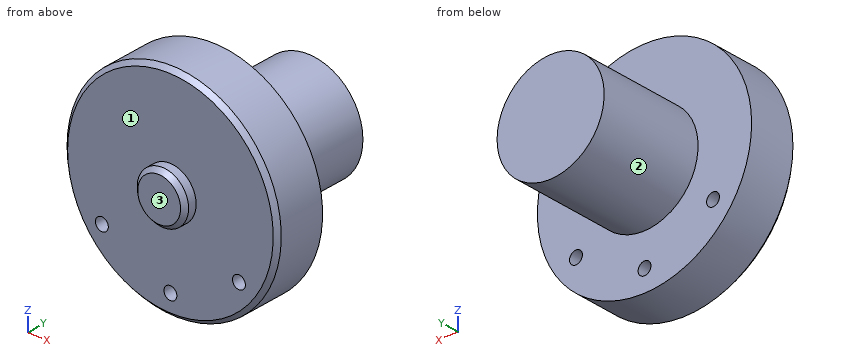
Autodesk Inventor part; units mm, degrees
ref_plane "YZ Plane" through (0, 0, 0) normal (1, 0, 0) x (0, 1, 0)
ref_plane "XZ Plane" through (0, 0, 0) normal (0, 1, 0) x (-1, 0, 0)
ref_plane "XY Plane" through (0, 0, 0) normal (0, 0, 1) x (1, 0, 0)
sketch "Szkic1" plane through (0, 0, 0) normal (0, 1, 0) x (-1, 0, 0)
  circle A0 centre (0, 0) radius 25
  dimension "d0" = 50
extrude "Wyciągnięcie proste1" add sketch "Szkic1" along normal blind 12
sketch "Szkic2" plane through (0, 0, 0) normal (0, -1, 0) x (1, 0, 0)
  circle A0 centre (0, 0) radius 6
  dimension "d3" = 12
extrude "Wyciągnięcie proste2" add sketch "Szkic2" along normal blind 3
sketch "Szkic3" plane through (0, 12, 0) normal (0, 1, 0) x (1, 0, 0)
  circle A0 centre (0, 0) radius 12.5
  dimension "d6" = 25
extrude "Wyciągnięcie proste3" add sketch "Szkic3" along normal blind 25
chamfer "Faza1" distance 1 angle 45 1 edges at (-6, -3, 0)
chamfer "Faza2" distance 1 angle 45 1 edges at (25, 0, 0)
sketch "Szkic6" plane through (0, 0, 0) normal (0, -1, 0) x (1, 0, 0)
  circle A0 centre (0, 0) radius 20
  circle A1 centre (-16, -12) radius 1.5
  dimension "d16" = 40
  dimension "d17" = 3
extrude "Wyciągnięcie proste4" cut sketch "Szkic6" against normal blind 25 contours A1 A0 | A0 A1 picked at (-15.6226, -11.6657) picked at (-16.3566, -12.3446)
sketch "Szkic7" plane through (0, 0, 0) normal (0, -1, 0) x (1, 0, 0)
  circle A0 centre (0, 0) radius 5
  circle A1 centre (0, 0) radius 20
  circle A2 centre (16, -12) radius 1.5
  dimension "d20" = 40
  dimension "d21" = 3
extrude "Wyciągnięcie proste5" cut sketch "Szkic7" against normal blind 25 contours A2 A1 | A1 A2 picked at (15.5641, -11.7467) picked at (16.3868, -12.3102)
sketch "Szkic9" plane through (0, 0, 0) normal (0, -1, 0) x (1, 0, 0)
  circle A0 centre (0, -20) radius 1.5
  point P0 (0, 0)
  dimension "d25" = 3
extrude "Wyciągnięcie proste6" cut sketch "Szkic9" against normal blind 25
The listing builds one solid part. Answer for the finished solid, in the listing's coordinates (mm). Face numbers are marked on the shaded views. A direction names the side the tool comes from. Round coordinates to 2 decimals unless told otherwise and drop trailing zeros. Loops run counter-clockwise (first coordinate to the right, second up) from the corner with the lowest first, then second, coordinate; pieces in that order, holes last.
Q1. Given pin 1 Ø10 at (x, z) = (10, -16.5) entering from +Y; pin 2 Ø24 at (x, z) = (-5.5, -9.5) entering from -Y; pin 3 Ø8 at (x, y) = (-10, 22.5) entering from -Z; pin 4 Ø3 at (x, z) = (-1.5, -8) entering from -Y, each flat-ended and moving along its own axis, determine where each tip first touches the part or whether it passes through.
Q2. Find the intervals of material crossed by line 1 (Z direction, x = 0, y = 8); line 2 (X direction, y = 8, z = -12); line 3 (Y direction, x = -13.5, z = 0.5), in increasing order.
Q3. Section B-B, the plane z = 0 is taken. Determine the outline of the cut face in (x, y).
Q4. Section C-C, the plane y = 5 is taken. Determine the outline of the cut face in (x, z), then the cut area to 3 significant figures.
Q5. Section A-A, the plane x = 0 is taken. Determine the outline of the cut face in (y, z), then the cut area to 3 significant figures.
Q6. Which of the six approach directions +Z, -Z, +X, -X, +Y, -Y give full straight-line access (tool end or side, diameter ignored) to the marked faces 1, 2 and 3?
Q7. Section D-D, the plane y = 17 is taken. Determine the outline of the cut face in (x, z).
Completed:
1. pin 1: stops at y = 12
1. pin 2: stops at y = -3
1. pin 3: stops at z = -10.97
1. pin 4: stops at y = 0
2. line 1: z = -25 to -21.5, -18.5 to 25
2. line 2: x = -21.93 to -17.5, -14.5 to 14.5, 17.5 to 21.93
2. line 3: y = 0 to 12
3. outline: (-25, 1) - (-24, 0) - (-6, 0) - (-6, -2) - (-5, -3) - (5, -3) - (6, -2) - (6, 0) - (24, 0) - (25, 1) - (25, 12) - (12.5, 12) - (12.5, 37) - (-12.5, 37) - (-12.5, 12) - (-25, 12) - close
4. outline: circle Ø50 at (0, 0); hole circle Ø3 at (-16, -12); hole circle Ø3 at (0, -20); hole circle Ø3 at (16, -12)
4. area: 1,940 mm2
5. outline: (-3, -5) - (-2, -6) - (0, -6) - (0, -18.5) - (12, -18.5) - (12, -12.5) - (37, -12.5) - (37, 12.5) - (12, 12.5) - (12, 25) - (1, 25) - (0, 24) - (0, 6) - (-2, 6) - (-3, 5) - close; (0, -24) - (1, -25) - (12, -25) - (12, -21.5) - (0, -21.5) - close
5. area: 1,220 mm2
6. face 1: -Y
6. face 2: +Y
6. face 3: +Z, -Z, +X, -X, -Y
7. outline: circle Ø25 at (0, 0)
